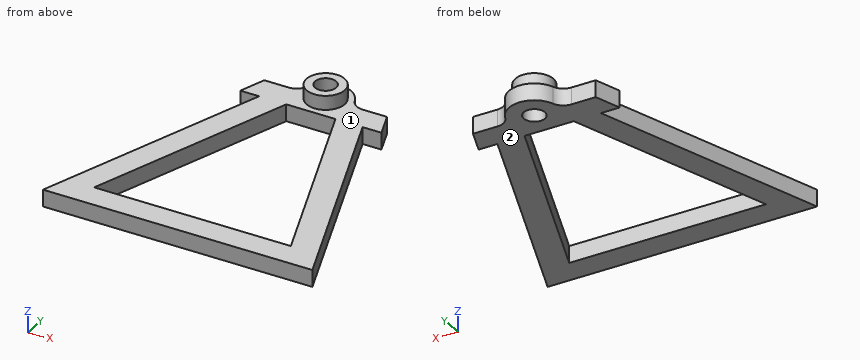
from build123d import *

# Parameters (mm, degrees)
F1_DEPTH = 0.6096
F2_R     = 0.381
F3_DEPTH = 25.4
F4_R     = 0.508
F5_R     = 0.6858
F5_R_2   = 0.381
F6_DEPTH = 0.508


with BuildPart() as f1:
    # F0 (on Top) → F1 (new body)
    with BuildSketch(Plane.XY):
        with BuildLine():
            Line((-1.8542, 8.2296), (-4.826, 0))
            Line((-4.826, 0), (0, 0))
            Line((0, 0), (4.826, 0))
            Line((4.826, 0), (1.8542, 8.2296))
            Line((1.8542, 8.2296), (2.528635, 8.2296))
            Line((2.528635, 8.2296), (2.198435, 9.144))
            Line((2.198435, 9.144), (1.524, 9.144))
            Line((1.524, 9.144), (0.9144, 9.144))
            ThreePointArc((0.9144, 9.144), (0, 10.0584), (-0.9144, 9.144))
            Line((-0.9144, 9.144), (-1.524, 9.144))
            Line((-1.524, 9.144), (-2.198435, 9.144))
            Line((-2.198435, 9.144), (-2.528635, 8.2296))
            Line((-2.528635, 8.2296), (-1.8542, 8.2296))
        make_face()
        Polygon((3.523607, 0.9144), (0, 0.9144), (-3.523607, 0.9144), (-0.882007, 8.2296), (0, 8.2296), (0.882007, 8.2296), align=None, mode=Mode.SUBTRACT)
    extrude(amount=F1_DEPTH)

    # F2 (on face) → F3 (cut)
    with BuildSketch(Plane.XY.offset(0.6096)):
        with Locations((0, 9.144)):
            Circle(F2_R)
    extrude(amount=-F3_DEPTH, mode=Mode.SUBTRACT)

    # F4
    f4_edges = [f1.edges().sort_by_distance(p)[0] for p in [
        (0.9144, 9.144, 0.3048),
        (-0.9144, 9.144, 0.3048),
    ]]
    fillet(f4_edges, radius=F4_R)

    # F5 (on face) → F6 (join)
    with BuildSketch(Plane.XY.offset(0.6096)):
        with Locations((0, 9.144)):
            Circle(F5_R)
        with Locations((0, 9.144)):
            Circle(F5_R_2, mode=Mode.SUBTRACT)
    extrude(amount=F6_DEPTH)


solid = f1.part
Can you work these out from the model? Positions are in its coordinate system, mm. Face numbers are marked on the shaded views. Coordinates: 2 decimals unless noted, no trailing zeros. Write each loop counter-clockwise with the first axis right and the second up, starting at its lowest first coordinate (ties: lowest second). Pieces come first, ordered by that corner, then holes. Notation, with made-up numbers: (63, -6.75) -> (104, -6.75) arc R34 cw to (104, 25.25) -> close; hole circle Ø2 at (2, 35). An arc over 180 degrees is marked (long way). Write item = value, one per line.
(1) If I drill on probe 1 along Y at (x, z) = (0, 0.2) (3 decimals); probe 2 along Y at (x, z) = (0, 0.95) (3 decimals); probe 3 along Y at (x, z) = (-0.25, 0.5), over which ranges is the centre line in solid material (lowest first)?
Verdict:
probe_1 = 0 to 0.914, 8.23 to 8.763, 9.525 to 10.058
probe_2 = 8.458 to 8.763, 9.525 to 9.83
probe_3 = 0 to 0.91, 8.23 to 8.86, 9.43 to 10.02
(2) Imagine slicing it at C-C (x = 2.75). Please give me the cut outline in (y, z), and give its area (3 significant figures).
Verdict:
outline = (0, 0) -> (0.91, 0) -> (0.91, 0.61) -> (0, 0.61) -> close; (3.06, 0) -> (5.75, 0) -> (5.75, 0.61) -> (3.06, 0.61) -> close
area = 2.20 mm^2
(3) For pin 1 (0.5 mm diameter, centred on x = -1.5, z = 0, fed in from +Y), with a flat end and sliding along its axis, tell me the tip position at first contact or that it passes through.
Verdict:
pin_1 = 9.15
(4) Thinking about a two-plate mould opening in Z: for the marked faces 1 and 2, which applies, +Z half, -Z half, draft (parallel to the pull), parting line (faces both ways), or undercut?
Verdict:
face_1 = +Z half
face_2 = -Z half
(5) Imagine slicing it at D-D (z = 0.8). Please give me the cut outline in (x, y), and give its area (3 significant figures).
Verdict:
outline = circle Ø1.37 at (0, 9.14); hole circle Ø0.76 at (0, 9.14)
area = 1.02 mm^2
(6) Imagine slicing it at B-B (y = 7.75). Please give me the cut outline in (x, z), and give its area (3 significant figures).
Verdict:
outline = (-2.03, 0) -> (-1.06, 0) -> (-1.06, 0.61) -> (-2.03, 0.61) -> close; (1.06, 0) -> (2.03, 0) -> (2.03, 0.61) -> (1.06, 0.61) -> close
area = 1.19 mm^2
(7) Imagine slicing it at A-A (x = 0). Please give me the cut outline in (y, z) (3 decimals).
Verdict:
outline = (0, 0) -> (0.914, 0) -> (0.914, 0.61) -> (0, 0.61) -> close; (8.23, 0) -> (8.763, 0) -> (8.763, 1.118) -> (8.458, 1.118) -> (8.458, 0.61) -> (8.23, 0.61) -> close; (9.525, 0) -> (10.058, 0) -> (10.058, 0.61) -> (9.83, 0.61) -> (9.83, 1.118) -> (9.525, 1.118) -> close
